Design review of the part built by this model. Coordinates are the model's own, in mm. Coordinates: 2 decimals unless noted, no trailing zeros. Loops run counter-clockwise (first coordinate to the right, second up) from the corner with the lowest first, then second, coordinate; pieces in that order, holes last.
Q1. Add section A-A on z = 11.25. Give the boundary of the cut face in (x, y).
Q2. Wall thickness on probe 1 along X at (y, z) = (23.5, 2); probe 2 along X at (y, z) = (26, 3.75); probe 3 along Y at (x, z) = (33, 4.75): over which ranges is each line inside the solid? List them lowest first.
Q3. Add section C-C on y = 28. Give the boundary of the cut face in (x, z).
Q4. Add section B-B on y = -28.5. Give the boundary of the cut face in (x, z).
Q5. For P1, Ø1.5, axis at x = -18, y = -17.5, coming from the -Z side, flat-tipped, find the tip position at first contact; note if it passes through.
```python
from build123d import *

# Parameters (mm, degrees)
F0_W     = 76.2
F0_H     = 76.2
F1_DEPTH = 12.7
F2_SIZE  = 12.7
F3_R     = 5.08


with BuildPart() as f1:
    # F0 (on Top) → F1 (new body)
    with BuildSketch(Plane.XY):
        Rectangle(F0_W, F0_H)
    extrude(amount=F1_DEPTH)

    # F2
    f2_edges = [f1.edges().sort_by_distance(p)[0] for p in [
        (-38.1, -38.1, 6.35),
        (38.1, -38.1, 6.35),
        (-38.1, 38.1, 6.35),
        (38.1, 38.1, 6.35),
    ]]
    chamfer(f2_edges, length=F2_SIZE)

    # F3
    f3_edges = [f1.edges().sort_by_distance(p)[0] for p in [
        (25.4, -38.1, 6.35),
        (38.1, -25.4, 6.35),
        (38.1, 25.4, 6.35),
        (25.4, 38.1, 6.35),
        (-25.4, 38.1, 6.35),
        (-38.1, 25.4, 6.35),
        (-38.1, -25.4, 6.35),
        (-25.4, -38.1, 6.35),
    ]]
    fillet(f3_edges, radius=F3_R)


solid = f1.part
```
Entries:
1. outline: (-38.1, -23.3) arc R5.08 ccw to (-36.61, -26.89) - (-26.89, -36.61) arc R5.08 ccw to (-23.3, -38.1) - (23.3, -38.1) arc R5.08 ccw to (26.89, -36.61) - (36.61, -26.89) arc R5.08 ccw to (38.1, -23.3) - (38.1, 23.3) arc R5.08 ccw to (36.61, 26.89) - (26.89, 36.61) arc R5.08 ccw to (23.3, 38.1) - (-23.3, 38.1) arc R5.08 ccw to (-26.89, 36.61) - (-36.61, 26.89) arc R5.08 ccw to (-38.1, 23.3) - close
2. probe 1: x = -38.1 to 38.1
2. probe 2: x = -37.32 to 37.32
2. probe 3: y = -30.5 to 30.5
3. outline: (-35.5, 0) - (35.5, 0) - (35.5, 12.7) - (-35.5, 12.7) - close
4. outline: (-35, 0) - (35, 0) - (35, 12.7) - (-35, 12.7) - close
5. P1: stops at z = 0
